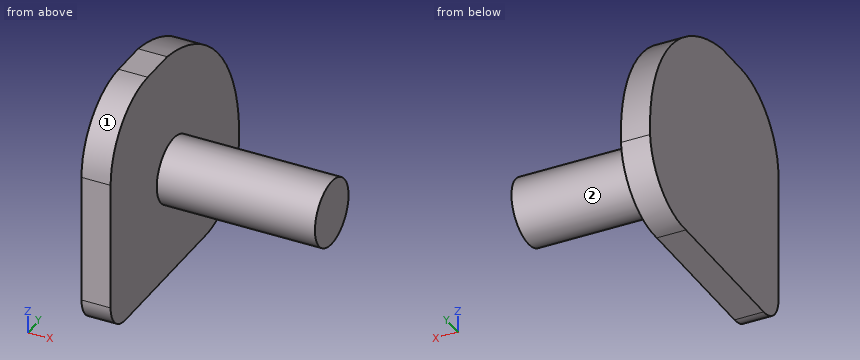
```python
from build123d import *

# Parameters (mm, degrees)
BOSS_EXTRUDE1_DEPTH = 20
SCALE1_SCALE        = 0.110510806
SKETCH4_R           = 2.5
BOSS_EXTRUDE2_DEPTH = 12


with BuildPart() as part:
    # Sketch3 → Boss-Extrude1 (new body)
    with BuildSketch(Plane(origin=(0, 0, 0), x_dir=(0, 0, -1), z_dir=(1, 0, 0))):
        with BuildLine():
            Line((0, -60), (0, -86.184781703))
            ThreePointArc((0, -86.184781703), (14.644660941, -121.540120762), (50, -136.184781703))
            Line((50, -136.184781703), (59.297038535, -136.184781703))
            Line((59.297038535, -136.184781703), (138.939006392, -136.184781703))
            ThreePointArc((138.939006392, -136.184781703), (153.081142016, -130.326917326), (158.939006392, -116.184781703))
            Line((158.939006392, -116.184781703), (158.939006392, -50))
            Line((158.939006392, -50), (158.939006392, -11.480346054))
            ThreePointArc((158.939006392, -11.480346054), (148.053108697, 21.328755123), (117.156078712, 36.830801017))
            ThreePointArc((117.156078712, 36.830801017), (39.60735059, 11.368133348), (0, -60))
        make_face()
    extrude(amount=BOSS_EXTRUDE1_DEPTH)


with BuildPart() as part_1:
    # Scale1: scaled about (10, -55.771836123, -85.371281571)
    add(part.part.scale(SCALE1_SCALE).moved(Location((8.89489194, -49.608445561, -75.936832435))))

    # Sketch4 → Boss-Extrude2 (add)
    with BuildSketch(Plane(origin=(11.10510806, 0, 0), x_dir=(0, 0, -1), z_dir=(1, 0, 0))):
        with Locations((85.501310137, -55.288244055)):
            Circle(SKETCH4_R)
    extrude(amount=BOSS_EXTRUDE2_DEPTH)


solid = part_1.part
```
Geometry check sheet. Reference: the model listing, model coordinates, mm. Face numbers are marked on the shaded views. A direction names the side the tool comes from. Coordinates: 2 decimals unless noted, no trailing zeros. Loops run counter-clockwise (first coordinate to the right, second up) from the corner with the lowest first, then second, coordinate; pieces in that order, holes last.
Item 1: Sectioned sample at B-B, the plane z = -85.75. Record the boundary of the cut face in (x, y).
Item 2: Access from +Z, -Z, +X, -X, +Y, -Y to the whole of each face (thin tool, end or side, straight path). Record for the marked faces 1 and 2.
Item 3: Thickness scan on line 1 (X direction, y = -53, z = -87.75); line 2 (Y direction, x = 10, z = -89.25); line 3 (Z direction, x = 20.25, y = -57). Record the ranges inside material, lowest first.
Item 4: Sectioned sample at A-A, the plane x = 10. Record the boundary of the cut face in (y, z).
Item 5: Go/stop test with flat-tipped pins: pin 1 Ø3 at (x, y) = (21.5, -51.5) entering from -Z; pin 2 Ø6 at (x, y) = (17.5, -51) entering from -Z; pin 3 Ø6 at (y, z) = (-48.5, -83) entering from +X. Record where each tip stops, or that it passes through.
Item 6: Sectioned sample at D-D, the plane y = -58.5. Record the boundary of the cut face in (x, z), then the cut area to 3 significant figures.
Item 7: Sectioned sample at C-C, the plane y = -55. Record the boundary of the cut face in (x, z), then the cut area to 3 significant figures.
Check result:
1. outline: (8.89, -64.66) - (11.11, -64.66) - (11.11, -57.78) - (23.11, -57.78) - (23.11, -52.8) - (11.11, -52.8) - (11.11, -45.76) - (8.89, -45.76) - close
2. face 1: +Z, +X, -X, -Y
2. face 2: +X
3. line 1: x = 8.89 to 11.11
3. line 2: y = -64.66 to -45.58
3. line 3: z = -87.32 to -83.68
4. outline: (-64.66, -91.29) arc R2.21 ccw to (-62.45, -93.5) - (-50.88, -93.5) arc R4.99 ccw to (-45.54, -88.88) arc R12.36 ccw to (-56.24, -75.94) - (-59.13, -75.94) arc R5.53 ccw to (-64.66, -81.46) - close
5. pin 1: stops at z = -86.51
5. pin 2: stops at z = -87.64
5. pin 3: stops at x = 11.11
6. outline: (8.89, -93.5) - (11.11, -93.5) - (11.11, -75.94) - (8.89, -75.94) - close
6. area: 38.8 mm2
7. outline: (8.89, -93.5) - (11.11, -93.5) - (11.11, -87.98) - (23.11, -87.98) - (23.11, -83.02) - (11.11, -83.02) - (11.11, -76.17) - (8.89, -76.17) - close
7. area: 97.9 mm2
